Read the model definition and answer for the solid it produces. Units are mm, in the model's axes. A direction names the side the tool comes from. Coordinates: 2 decimals unless noted, no trailing zeros. Write each loop counter-clockwise with the first axis right and the second up, starting at its lowest first coordinate (ties: lowest second). Pieces come first, ordered by that corner, then holes. Notation, with made-up numbers: (-37.5, 76) -> (6.5, 76) arc R12 ccw to (6.5, 93) -> close; hole circle Ø7 at (-19.75, 25.25). An arc over 180 degrees is marked (long way). Answer in a Markdown table with one row per item. Add a question column.
Item 1: Which of the six approach directions +Z, -Z, +X, -X, +Y, -Y give full straight-line access (tool end or side, diameter ignored) to faces 1 (the face through (28.18, 16.52, 4.42)), 2 (the face through (0, 31.75, 3)), 3 (the face through (-26.9, 17, 0)), 4 (the face through (-17.5, 17, -3))?
Item 2: Section A-A on y = 6.5 is taken. Write down the section's boundary in (x, z), then the cut area to 3 significant figures.
Item 3: Section B-B on x = 0 is taken. Write down the section's boundary in (y, z).
Item 4: Section C-C on z = 0.75 is taken. Write down the section's boundary in (x, y), then the cut area to 3 significant figures.
Item 5: Given pin 1 Ø5 at (y, z) = (16.5, -0.5) entering from +X; pin 2 Ø3 at (x, z) = (0, 0) entering from -Y; pin 3 Ø1.5 at (y, z) = (7, -1) entering from -X; pin 4 Ø4.5 at (y, z) = (16, -2.5) entering from -X, each flat-ended and moving along its own axis, determine where each tip first touches the part or whether it passes through.
Item 6: Section D-D on x = 7 is taken. Write down the section's boundary in (y, z).
Item 7: Straight lines are drawn through the part: line 1 (Y direction, x = 2, z = -4.25); line 2 (X direction, y = 8.5, z = -3); line 3 (X direction, y = 32.85, z = 0). For each, find the intervals that lie inside material, in ascending order. Write a range as from..to.
Item 8: For a pull along Y with two mould halves and no side action, classify faces 5 (the face through (-28.18, 16.52, -4.42)), 6 (the face through (0, 33.5, 3)), 7 (the face through (0, 1.75, 3)) as +Y half, -Y half, draft (parallel to the pull), parting line (faces both ways), or undercut.
Autodesk Inventor part; units mm, degrees
ref_plane "YZ Plane" through (0, 0, 0) normal (1, 0, 0) x (0, 1, 0)
ref_plane "XZ Plane" through (0, 0, 0) normal (0, 1, 0) x (-1, 0, 0)
ref_plane "XY Plane" through (0, 0, 0) normal (0, 0, 1) x (1, 0, 0)
sketch "Sketch1" plane through (0, 0, 0) normal (0, 1, 0) x (-1, 0, 0)
  line L0 (41.2832, 0) -> (-41.2832, 0) construction
  line L1 (0, -8.0192) -> (0, 8.0192) construction
  line L2 (26.9, 0) -> (26.9, -3.14)
  line L3 (26.9, -3.14) -> (29.488, -5.728)
  line L4 (29.488, -5.728) -> (0, -5.728)
  line L5 (26.9, 0) -> (26.9, 3.14)
  line L6 (26.9, 3.14) -> (29.488, 5.728)
  line L7 (29.488, 5.728) -> (0, 5.728)
  line L8 (-26.9, 0) -> (-26.9, -3.14)
  line L9 (-26.9, -3.14) -> (-29.488, -5.728)
  line L10 (-29.488, -5.728) -> (0, -5.728)
  line L11 (-26.9, 0) -> (-26.9, 3.14)
  line L12 (-26.9, 3.14) -> (-29.488, 5.728)
  line L13 (-29.488, 5.728) -> (0, 5.728)
  point P0 (0, 0)
  dimension "d0" = 26.9
  dimension "d1" = 3.14
  dimension "d2" = 3.66
  dimension "d3" = 135
extrude "Extrusion1" add sketch "Sketch1" along normal blind 33.5
sketch "Sketch2" plane through (-29.488, 0, 5.728) normal (0, 0, 1) x (1, 0, 0)
  line L0 (58.976, 0) -> (0, 0) construction
  line L1 (58.976, 0) -> (58.976, 33.5) construction
  line L2 (0, 33.5) -> (58.976, 33.5) construction
  line L3 (0, 0) -> (0, 33.5) construction
  line L4 (29.488, -6.8) -> (29.488, 40.8) construction
  line L5 (46.988, 1.75) -> (11.988, 1.75)
  line L6 (11.988, 1.75) -> (11.988, 31.75)
  line L7 (11.988, 31.75) -> (46.988, 31.75)
  line L8 (46.988, 31.75) -> (46.988, 1.75)
  line L9 (46.988, 1.75) -> (11.988, 31.75) construction
  line L10 (11.988, 1.75) -> (46.988, 31.75) construction
  point P0 (29.488, 16.75)
  dimension "d16" = 30
  dimension "d17" = 35
  dimension "d18" = 16.75
extrude "Extrusion2" cut sketch "Sketch2" against normal through all
sketch "Sketch3" plane through (0, 33.5, 0) normal (0, 1, 0) x (1, 0, 0)
  line L0 (-26.9, 3.14) -> (-26.9, -3.14) construction
  line L1 (-26.9, -3.14) -> (-29.488, -5.728) construction
  line L2 (-29.488, -5.728) -> (29.488, -5.728) construction
  line L3 (29.488, -5.728) -> (26.9, -3.14) construction
  line L4 (26.9, -3.14) -> (26.9, 3.14) construction
  line L5 (26.9, 3.14) -> (29.488, 5.728) construction
  line L6 (29.488, 5.728) -> (-29.488, 5.728) construction
  line L7 (-29.488, 5.728) -> (-26.9, 3.14) construction
  circle A0 centre (0, 0) radius 1.7
  dimension "d10" = 3.4
extrude "Extrusion3" cut sketch "Sketch3" against normal through all
ref_plane "Work Plane1" through (0, 29.5, 5.728) normal (0, -1, 0) x (1, 0, 0)
sketch "Sketch4" plane through (0, 29.5, 5.728) normal (0, -1, 0) x (1, 0, 0)
  circle A0 centre (0, -5.728) radius 1.7 construction
  line L0 (-26.9, -8.868) -> (-26.9, -2.588) construction
  line L1 (-26.9, -2.588) -> (-29.488, 0) construction
  line L2 (-29.488, 0) -> (29.488, 0) construction
  line L3 (29.488, 0) -> (26.9, -2.588) construction
  line L4 (26.9, -2.588) -> (26.9, -8.868) construction
  line L5 (26.9, -8.868) -> (29.488, -11.456) construction
  line L6 (29.488, -11.456) -> (-29.488, -11.456) construction
  line L7 (-29.488, -11.456) -> (-26.9, -8.868) construction
  line L8 (12.5, 0) -> (12.5, -11.456) construction
  line L9 (-12.5, 0) -> (-12.5, -11.456) construction
  line L10 (0, -5.728) -> (21.3772, 0)
  line L11 (0, -5.728) -> (22.1313, -5.728) construction
  line L12 (0, -13.7472) -> (0, 2.2912) construction
  line L13 (0, -5.728) -> (-21.3772, 0)
  line L14 (-21.3772, 0) -> (21.3772, 0)
  line L15 (29.488, 0) -> (-29.488, 0) construction
  dimension "d13" = 15
extrude "Extrusion4" [suppressed]
chamfer "Chamfer1" distance 10 angle 30 2 edges at (-17.5, 16.75, 5.728) (17.5, 16.75, 5.728) measured on face at (25.492, 11.75, 5.728)
Results below:
| question | item | result |
|---|---|---|
| 1 | face 1 | +X, +Y, -Y |
| 1 | face 2 | +Z |
| 1 | face 3 | -X, +Y, -Y |
| 1 | face 4 | +Z, -Z |
| 2 | outline | (-29.49, -5.73) -> (-17.5, -5.73) -> (-17.5, -0.05) -> (-27.5, 5.73) -> (-29.49, 5.73) -> (-26.9, 3.14) -> (-26.9, -3.14) -> close; (17.5, -5.73) -> (29.49, -5.73) -> (26.9, -3.14) -> (26.9, 3.14) -> (29.49, 5.73) -> (27.5, 5.73) -> (17.5, -0.05) -> close |
| 2 | area | 171 mm2 |
| 3 | outline | (0, -5.73) -> (1.75, -5.73) -> (1.75, -1.7) -> (0, -1.7) -> close; (0, 1.7) -> (1.75, 1.7) -> (1.75, 5.73) -> (0, 5.73) -> close; (31.75, -5.73) -> (33.5, -5.73) -> (33.5, -1.7) -> (31.75, -1.7) -> close; (31.75, 1.7) -> (33.5, 1.7) -> (33.5, 5.73) -> (31.75, 5.73) -> close |
| 4 | outline | (-26.9, 0) -> (-1.53, 0) -> (-1.53, 1.75) -> (-18.88, 1.75) -> (-18.88, 31.75) -> (-1.53, 31.75) -> (-1.53, 33.5) -> (-26.9, 33.5) -> close; (1.53, 0) -> (26.9, 0) -> (26.9, 33.5) -> (1.53, 33.5) -> (1.53, 31.75) -> (18.88, 31.75) -> (18.88, 1.75) -> (1.53, 1.75) -> close |
| 4 | area | 659 mm2 |
| 5 | pin 1 | stops at x = 26.9 |
| 5 | pin 2 | passes through |
| 5 | pin 3 | stops at x = -26.9 |
| 5 | pin 4 | stops at x = -28.51 |
| 6 | outline | (0, -5.73) -> (1.75, -5.73) -> (1.75, 5.73) -> (0, 5.73) -> close; (31.75, -5.73) -> (33.5, -5.73) -> (33.5, 5.73) -> (31.75, 5.73) -> close |
| 7 | line 1 | y = 0..1.75, 31.75..33.5 |
| 7 | line 2 | x = -26.9..-17.5, 17.5..26.9 |
| 7 | line 3 | x = -26.9..-1.7, 1.7..26.9 |
| 8 | face 5 | draft |
| 8 | face 6 | +Y half |
| 8 | face 7 | undercut |
